```python
from build123d import *

# Parameters (mm, degrees)
F0_W     = 9.1
F0_H     = 5.2
F1_DEPTH = 14.6
F2_R     = 2.5
F3_W     = 6.7
F3_H     = 1.5
F4_DEPTH = 6.7
F5_R     = 0.5


with BuildPart() as f1:
    # F0 (on Front) → F1 (new body)
    with BuildSketch(Plane.XZ):
        with Locations((6.69256, 11.174007)):
            Rectangle(F0_W, F0_H)
    extrude(amount=F1_DEPTH)

    # F2
    f2_edges = [f1.edges().sort_by_distance(p)[0] for p in [
        (11.24256, -7.3, 8.574007),
        (11.24256, -7.3, 13.774007),
        (2.14256, -7.3, 8.574007),
        (2.14256, -7.3, 13.774007),
    ]]
    fillet(f2_edges, radius=F2_R)

    # F3 (on face) → F4 (join)
    with BuildSketch(Plane.XZ.offset(14.6)):
        with Locations((6.69256, 11.174007)):
            Rectangle(F3_W, F3_H)
    extrude(amount=F4_DEPTH)

    # F5
    f5_edges = [f1.edges().sort_by_distance(p)[0] for p in [
        (3.34256, -17.95, 10.424007),
        (10.04256, -17.95, 10.424007),
        (10.04256, -17.95, 11.924007),
        (3.34256, -17.95, 11.924007),
    ]]
    fillet(f5_edges, radius=F5_R)


solid = f1.part
```
Verification items for the finished model (mm, model axes). A direction names the side the tool comes from. Coordinates: 2 decimals unless noted, no trailing zeros. Write each loop counter-clockwise with the first axis right and the second up, starting at its lowest first coordinate (ties: lowest second). Pieces come first, ordered by that corner, then holes. Notation, with made-up numbers: M 15,-22.75 L 28,-22.75 A36 ccw 28,13.25 Z; hole C -16,22.5 d2. An arc over 180 degrees is marked long. One line per item, written item: value.
Item 1: Access from +Z, -Z, +X, -X, +Y, -Y to the whole of each face (thin tool, end or side, straight path). Record for faces 1 (the flat face through (7, -18, 10.424)), 2 (the flat face through (7, -21.3, 11)), 3 (the flat face through (7, -18, 11.924)).
Check sheet entries:
face 1: -Z, +X, -X, -Y
face 2: +Z, -Z, +X, -X, -Y
face 3: +Z, +X, -X, -Y
Item 2: Section check B-B, the plane y = -6.5. Record the boundary of the cut face in (x, z).
Check sheet entries:
outline: M 2.14,11.07 A2.5 ccw 4.64,8.57 L 8.74,8.57 A2.5 ccw 11.24,11.07 L 11.24,11.27 A2.5 ccw 8.74,13.77 L 4.64,13.77 A2.5 ccw 2.14,11.27 Z
Item 3: Section check D-D, the plane z = 9.9. Record the boundary of the cut face in (x, y), plus the area to 3 significant figures.
Check sheet entries:
outline: M 2.44,-14.6 L 10.95,-14.6 L 10.95,0 L 2.44,0 Z
area: 124 mm^2
Item 4: Section check A-A, the plane x = 6. Record the boundary of the cut face in (y, z), plus the area to 3 significant figures.
Check sheet entries:
outline: M -21.3,10.42 L -14.6,10.42 L -14.6,8.57 L 0,8.57 L 0,13.77 L -14.6,13.77 L -14.6,11.92 L -21.3,11.92 Z
area: 86.0 mm^2
Item 5: Scan lines: line 1 along Z through (x, y) = (4.5, -18.5); line 2 along Y through (x, z) = (10, 10.2); line 3 along X through (y, z) = (-4.25, 11.95). Record each from-to range of solid material in increasing order.
Check sheet entries:
line 1: z = 10.42 to 11.92
line 2: y = -14.6 to 0
line 3: x = 2.24 to 11.15
Item 6: Section check C-C, the plane z = 12.25. Record the boundary of the cut face in (x, y), plus the area to 3 significant figures.
Check sheet entries:
outline: M 2.34,-14.6 L 11.04,-14.6 L 11.04,0 L 2.34,0 Z
area: 127 mm^2
Item 7: Gauge pin test, flat ends, axial feed: pin 1 Ø4.5 at (x, y) = (7.5, -18.5) entering from +Z; pin 2 Ø4.5 at (x, y) = (7.5, -18) entering from -Z; pin 3 Ø1 at (x, z) = (9, 10.5) entering from +Y; pin 4 Ø0.6 at (y, z) = (-17, 11) entering from -X. Record the tip position at first contact, or that the pin passes through.
Check sheet entries:
pin 1: stops at z = 11.92
pin 2: stops at z = 10.42
pin 3: stops at y = 0
pin 4: stops at x = 3.34
